from build123d import *

# Parameters (mm, degrees)
SKETCH1_W            = 30
SKETCH1_H            = 40
BOSS_EXTRUDE1_DEPTH  = 15
CUT_EXTRUDE1_DEPTH   = 49
SKETCH3_R            = 1.5
CUT_EXTRUDE2_DEPTH   = 49
SKETCH4_R            = 1.75
BOSS_EXTRUDE2_DEPTH  = 28
SKETCH5_W            = 6
SKETCH5_H            = 35
BOSS_EXTRUDE3_DEPTH  = 9
SKETCH6_R            = 1.75
BOSS_EXTRUDE4_DEPTH  = 15
SKETCH7_W            = 15
SKETCH7_H            = 40
BOSS_EXTRUDE6_DEPTH  = 30
CUT_EXTRUDE3_DEPTH   = 59
SKETCH10_R           = 1.5
CUT_EXTRUDE4_DEPTH   = 59
SKETCH14_W           = 14
SKETCH14_H           = 15
BOSS_EXTRUDE8_DEPTH  = 15
CUT_EXTRUDE7_DEPTH   = 21
SKETCH17_W           = 9
SKETCH17_H           = 12
BOSS_EXTRUDE10_DEPTH = 18.07


with BuildPart() as part:
    # Sketch1 → Boss-Extrude1 (new body)
    with BuildSketch(Plane.XY):
        with Locations((15, 20)):
            Rectangle(SKETCH1_W, SKETCH1_H)
    extrude(amount=BOSS_EXTRUDE1_DEPTH)

    # Sketch2 → Cut-Extrude1 (cut)
    with BuildSketch(Plane(origin=(0, 40, 0), x_dir=(1, 0, 0), z_dir=(0, 1, 0))):
        with BuildLine():
            Line((7.5, -15), (22.5, -15))
            ThreePointArc((22.5, -15), (15, -7.5), (7.5, -15))
        make_face()
    extrude(amount=-CUT_EXTRUDE1_DEPTH, mode=Mode.SUBTRACT)

    # Sketch3 → Cut-Extrude2 (cut)
    with BuildSketch(Plane.XY.offset(15)):
        with Locations((3, 34)):
            Circle(SKETCH3_R)
        with Locations((3, 6)):
            Circle(SKETCH3_R)
        with Locations((27, 34)):
            Circle(SKETCH3_R)
        with Locations((27, 6)):
            Circle(SKETCH3_R)
    extrude(amount=-CUT_EXTRUDE2_DEPTH, mode=Mode.SUBTRACT)

    # Sketch4 → Boss-Extrude2 (add)
    with BuildSketch(Plane(origin=(30, 0, 0), x_dir=(0, 0, -1), z_dir=(1, 0, 0))):
        with Locations(Location((-3, 34, 0), (0, 0, 180))):
            Circle(SKETCH4_R)
        with Locations(Location((-3, 6, 0), (0, 0, 180))):
            Circle(SKETCH4_R)
    extrude(amount=BOSS_EXTRUDE2_DEPTH)

    # Sketch5 → Boss-Extrude3 (add)
    with BuildSketch(Plane(origin=(58, 0, 0), x_dir=(0, 0, -1), z_dir=(1, 0, 0))):
        with Locations((-3, 20)):
            Rectangle(SKETCH5_W, SKETCH5_H)
    extrude(amount=BOSS_EXTRUDE3_DEPTH)

    # Sketch6 → Boss-Extrude4 (add)
    with BuildSketch(Plane(origin=(67, 0, 0), x_dir=(0, 0, -1), z_dir=(1, 0, 0))):
        with Locations(Location((-3, 34, 0), (0, 0, 180))):
            Circle(SKETCH6_R)
        with Locations(Location((-3, 6, 0), (0, 0, 180))):
            Circle(SKETCH6_R)
    extrude(amount=BOSS_EXTRUDE4_DEPTH)

    # Sketch7 → Boss-Extrude6 (add)
    with BuildSketch(Plane(origin=(82, 0, 0), x_dir=(0, 0, -1), z_dir=(1, 0, 0))):
        with Locations((-7.5, 20)):
            Rectangle(SKETCH7_W, SKETCH7_H)
    extrude(amount=BOSS_EXTRUDE6_DEPTH)

    # Sketch9 → Cut-Extrude3 (cut)
    with BuildSketch(Plane(origin=(0, 40, 0), x_dir=(1, 0, 0), z_dir=(0, 1, 0))):
        with BuildLine():
            Line((89.5, -15), (104.5, -15))
            ThreePointArc((104.5, -15), (97, -7.5), (89.5, -15))
        make_face()
    extrude(amount=-CUT_EXTRUDE3_DEPTH, mode=Mode.SUBTRACT)

    # Sketch10 → Cut-Extrude4 (cut)
    with BuildSketch(Plane.XY.offset(15)):
        with Locations((85, 34)):
            Circle(SKETCH10_R)
        with Locations((109, 34)):
            Circle(SKETCH10_R)
        with Locations((109, 6)):
            Circle(SKETCH10_R)
        with Locations((85, 6)):
            Circle(SKETCH10_R)
    extrude(amount=-CUT_EXTRUDE4_DEPTH, mode=Mode.SUBTRACT)

    # Sketch14 → Boss-Extrude8 (add)
    with BuildSketch(Plane(origin=(0, 0, 0), x_dir=(-1, 0, 0), z_dir=(0, 0, -1))):
        with Locations((-97, 19.5)):
            Rectangle(SKETCH14_W, SKETCH14_H)
    boss_extrude8 = extrude(amount=BOSS_EXTRUDE8_DEPTH)

    # Sketch15 → Cut-Extrude7 (cut)
    with BuildSketch(Plane(origin=(104, 0, 0), x_dir=(0, 0, -1), z_dir=(1, 0, 0))):
        Polygon((0, 12), (15, 20.660254038), (15, 12), align=None)
    cut_extrude7 = extrude(amount=-CUT_EXTRUDE7_DEPTH, mode=Mode.SUBTRACT)

    # Mirror1: Boss-Extrude8, Cut-Extrude7 across plane
    add(boss_extrude8.mirror(Plane(origin=(56, 0, 0), x_dir=(0, 0, 1), z_dir=(1, 0, 0))))
    add(cut_extrude7.mirror(Plane(origin=(56, 0, 0), x_dir=(0, 0, 1), z_dir=(1, 0, 0))), mode=Mode.SUBTRACT)

    # Sketch17 → Boss-Extrude10 (add)
    with BuildSketch(Plane.XY.offset(6)):
        with Locations((62.5, 20.5)):
            Rectangle(SKETCH17_W, SKETCH17_H)
    extrude(amount=BOSS_EXTRUDE10_DEPTH)


solid = part.part
Geometry check sheet. Reference: the model listing, model coordinates, mm. A direction names the side the tool comes from. Coordinates: 2 decimals unless noted, no trailing zeros. Write each loop counter-clockwise with the first axis right and the second up, starting at its lowest first coordinate (ties: lowest second). Pieces come first, ordered by that corner, then holes. Notation, with made-up numbers: (-5, -3) -> (41, -3) arc R32 cw to (41, 35) -> close; hole circle Ø10 at (70, -8). An arc over 180 degrees is marked (long way). One line per question, with ' | ' between items.
1. Set-up check for faces 5 (the flat face through (104, 21, -6)), 6 (the flat face through (62, 32, 6)), 7 (the cylindrical face through (43.804, 33.474, 4.669)), 8 (the flat face through (62, 8, 6)), 9 (the flat face through (26, 20, 15)): record each of +Z, -Z, +X, -X, +Y, -Y from which the full face is reachable in a straight line by a thin tool's end or side.
Answers:
face 5: -Z, +X, +Y, -Y | face 6: +Z, +Y | face 7: none | face 8: +Z, -Y | face 9: +Z, -X, +Y, -Y
2. Cross-section at A-A on y = 9.5. Record the cut outline in (x, z), and give its area (3 significant figures).
Answers:
outline: (0, 0) -> (30, 0) -> (30, 15) -> (22.5, 15) arc R7.5 cw to (7.5, 15) -> (0, 15) -> close; (58, 0) -> (67, 0) -> (67, 6) -> (58, 6) -> close; (82, 0) -> (112, 0) -> (112, 15) -> (104.5, 15) arc R7.5 cw to (89.5, 15) -> (82, 15) -> close | area: 777 mm²
3. Cross-section at C-C on z = -7.5. Record the cut outline in (x, y).
Answers:
outline: (8, 16.33) -> (22, 16.33) -> (22, 27) -> (8, 27) -> close; (90, 16.33) -> (104, 16.33) -> (104, 27) -> (90, 27) -> close
4. Thickness scan on probe 1 along Y at (x, z) = (3, 10); probe 2 along X at (y, z) = (8, 2.5); probe 3 along X at (y, z) = (22.5, 9). Record the ranges inside material, lowest first. Write a range as from..to.
Answers:
probe 1: y = 0..4.5, 7.5..32.5, 35.5..40 | probe 2: x = 0..30, 58..67, 82..112 | probe 3: x = 0..10.5, 19.5..30, 58..67, 82..92.5, 101.5..112
5. Cross-section at B-B on x = 109. Record the cut outline in (y, z).
Answers:
outline: (0, 0) -> (4.5, 0) -> (4.5, 15) -> (0, 15) -> close; (7.5, 0) -> (32.5, 0) -> (32.5, 15) -> (7.5, 15) -> close; (35.5, 0) -> (40, 0) -> (40, 15) -> (35.5, 15) -> close
6. Cross-section at D-D on z = 3. State how many separate pieces and enclosed holes the cut face has, and give its area (3 significant figures).
Answers:
separate pieces: 1 | enclosed holes: 10 | area: 2,960 mm²
7. Draft check along Y on faces 1 (the cylindrical face through (74.4, 7.55, 3.81)), 2 (the flat face through (97, 29, 0)), 3 (the flat face through (14.902, 16.27, -7.395)), 4 (the flat face through (15, 40, 6)). Enter one of: +Y half, -Y half, draft (parallel to the pull), parting line (faces both ways), or undercut.
Answers:
face 1: undercut | face 2: draft | face 3: -Y half | face 4: +Y half
8. Depth check by flat-ended pin: pin 1 Ø2.5 at (x, y) = (109, 6) entering from -Z; pin 2 Ø10 at (x, y) = (61.5, 7) entering from +Z; pin 3 Ø7.5 at (y, z) = (18, -9) entering from -X; pin 4 Ø4.5 at (x, y) = (64, 14.5) entering from -Z. Enter the tip coordinate at first touch or a pass-through.
Answers:
pin 1: passes through | pin 2: stops at z = 6 | pin 3: stops at x = 8 | pin 4: stops at z = 0
